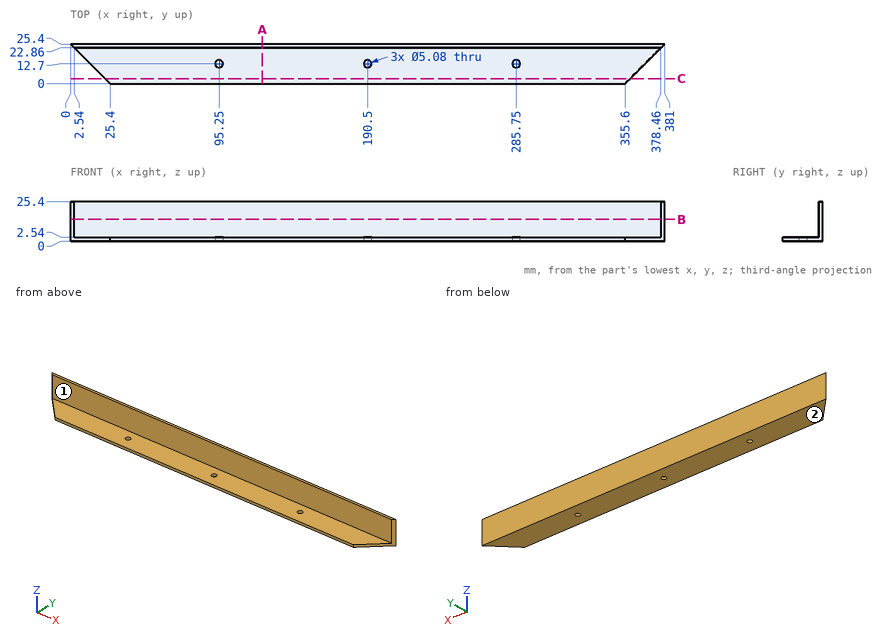
Could you check a few things on this drawing? It's one solid part, dimensions in mm from its lowest x, y, z. A direction names the side the tool comes from. Coordinates: 2 decimals unless noted, no trailing zeros. Write each loop counter-clockwise with the first axis right and the second up, starting at its lowest first coordinate (ties: lowest second). Pieces come first, ordered by that corner, then holes. Notation, with made-up numbers: (32, 49.25) - (56, 49.25) arc R26 cw to (56, 76.25) - close; hole circle Ø8 at (40.25, -23.75). An arc over 180 degrees is marked (long way). Put each result on its own line as item: value. Start each with the question number.
Q1. Which directions (+Z, -Z, +X, -X, +Y, -Y) give clear straight access to the entire face, cutting with the end or side of a thin tool? Please do the marked faces 1 and 2.
Q2. I want a section at A-A on x = 123. Write out the boundary of the cut face in (y, z).
Q3. I'm going to push flat-ended pins straight in: P1, Ø10, axis at y = 19, z = 17, coming from the +X side; P2, Ø4, axis at y = 22.5, z = 12, coming from the -X side; P3, Ø5, axis at x = 147, y = 11, coming from the +Z side. Where does each tip first touch, or does it pass through?
Q4. I want a section at C-C on y = 3.25. Write out the boundary of the cut face in (x, z).
Q5. Please list where these lines run through material, in increasing order: L1, parallel to Y at x = 190.5, z = 1.3; L2, parallel to Y at x = 359.5, z = 18.75; L3, parallel to Z at x = 104, y = 14.25.
Q6. I want a section at B-B on z = 14. Write out the boundary of the cut face in (x, y).
Checks:
1. face 1: +Z, +X, -X, -Y
1. face 2: -Z, +X, -X, +Y, -Y
2. outline: (0, 0) - (25.4, 0) - (25.4, 25.4) - (22.86, 25.4) - (22.86, 2.54) - (0, 2.54) - close
3. P1: x = 379.6
3. P2: x = 0.9
3. P3: z = 2.54
4. outline: (22.15, 0) - (358.85, 0) - (358.85, 2.54) - (22.15, 2.54) - close
5. L1: 0 to 10.16, 15.24 to 25.4
5. L2: 22.86 to 25.4
5. L3: 0 to 2.54
6. outline: (0, 25.4) - (2.54, 22.86) - (378.46, 22.86) - (381, 25.4) - close
